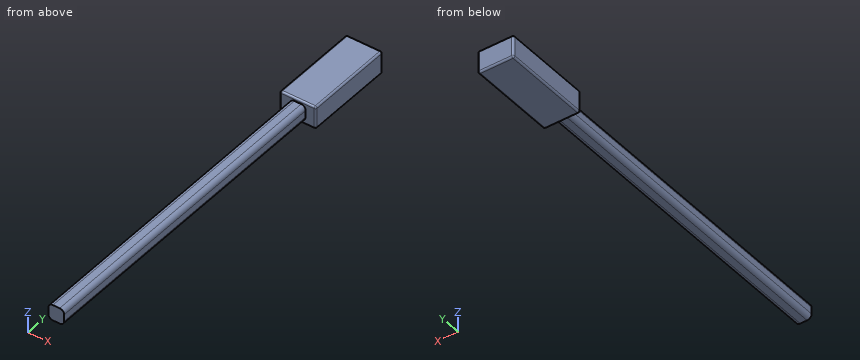
from build123d import *

# Parameters (mm, degrees)
F0_W     = 8
F0_H     = 20
F1_DEPTH = 2.5
F2_W     = 3.5
F2_H     = 75
F3_DEPTH = 1.75
F4_R     = 0.4
F5_R     = 1


with BuildPart() as f1:
    # F0 (on Top) → F1 (new body, symmetric)
    with BuildSketch(Plane.XY):
        Rectangle(F0_W, F0_H)
    extrude(amount=F1_DEPTH, both=True)

    # F2 (on Top) → F3 (join, symmetric)
    with BuildSketch(Plane.XY):
        with Locations((0, -44.9)):
            Rectangle(F2_W, F2_H)
    extrude(amount=F3_DEPTH, both=True)

    # F4
    f4_edges = [f1.edges().sort_by_distance(p)[0] for p in [
        (4, 10, 0),
        (0, 10, -2.5),
        (0, 10, 2.5),
        (-4, 0, 2.5),
        (4, 0, -2.5),
        (-4, 0, -2.5),
        (4, 0, 2.5),
        (-4, 10, 0),
        (4, -10, 0),
        (0, -10, 2.5),
        (-4, -10, 0),
        (0, -10, -2.5),
    ]]
    fillet(f4_edges, radius=F4_R)

    # F5
    f5_edges = [f1.edges().sort_by_distance(p)[0] for p in [
        (1.75, -46.2, -1.75),
        (-1.75, -46.2, -1.75),
        (1.75, -46.2, 1.75),
        (-1.75, -46.2, 1.75),
    ]]
    fillet(f5_edges, radius=F5_R)


solid = f1.part
Check sheet for the modelled part. Datum: model origin and axes. Units: mm. Round coordinates to 2 decimals unless told otherwise and drop trailing zeros. Loops run counter-clockwise (first coordinate to the right, second up) from the corner with the lowest first, then second, coordinate; pieces in that order, holes last. Notation, with made-up numbers: (56.5, 47) - (69.5, 47) arc R28 ccw to (69.5, 78) - close; hole circle Ø9 at (-24.5, -33.75). An arc over 180 degrees is marked (long way). Answer as CSV lines item,"result". Start each with the question number.
Item 1: Depth check by flat-ended pin: P1, Ø1.7, axis at x = 0.5, y = -35, coming from the +Z side; P2, Ø0.8, axis at y = -62, z = 0, coming from the -X side; P3, Ø1, axis at y = -31, z = 1.5, coming from the -X side. Enter the tip coordinate at first touch or a pass-through.
Item 2: Scan lines: line 1 (Y direction, x = -3.5, z = 1.3); line 2 (X direction, y = -55, z = -0.7); line 3 (X direction, y = -40, z = 0.9). Record each from-to range of solid material in increasing order. Write a range as [from, to].
Item 3: Section check B-B (y = -75). Record the boundary of the cut face in (x, z), and give its area (3 significant figures).
Item 4: Section check A-A (x = 0). Record the boundary of the cut face in (y, z), and give its area (3 significant figures).
Report:
1,P1,"stops at z = 1.75"
1,P2,"stops at x = -1.75"
1,P3,"stops at x = -1.72"
2,line 1,"y = [-10, 10]"
2,line 2,"x = [-1.75, 1.75]"
2,line 3,"x = [-1.74, 1.74]"
3,outline,"(-1.75, -0.75) arc R1 ccw to (-0.75, -1.75) - (0.75, -1.75) arc R1 ccw to (1.75, -0.75) - (1.75, 0.75) arc R1 ccw to (0.75, 1.75) - (-0.75, 1.75) arc R1 ccw to (-1.75, 0.75) - close"
3,area,"11.4 mm2"
4,outline,"(-82.4, -1.75) - (-10, -1.75) - (-10, -2.1) arc R0.4 ccw to (-9.6, -2.5) - (9.6, -2.5) arc R0.4 ccw to (10, -2.1) - (10, 2.1) arc R0.4 ccw to (9.6, 2.5) - (-9.6, 2.5) arc R0.4 ccw to (-10, 2.1) - (-10, 1.75) - (-82.4, 1.75) - close"
4,area,"353 mm2"
